```python
from build123d import *

# Parameters (mm, degrees)
F1_DEPTH = 1.5
F2_DEPTH = 14
F4_W     = 30
F4_H     = 17.707149
F5_DEPTH = 26
F6_R     = 3
F7_R     = 1
F9_DEPTH = 21.8


with BuildPart() as f1:
    # F0 (on Top) → F1 (new body)
    with BuildSketch(Plane.XY):
        Polygon((0, -20.207259), (17.5, -10.10363), (17.5, 10.10363), (0, 20.207259), (-17.5, 10.10363), (-17.5, -10.10363), align=None)
        with BuildLine():
            ThreePointArc((-6.29325, -8.626703), (-8.626703, -8.626703), (-8.626703, -6.29325))
            Line((-8.626703, -6.29325), (-6.434672, -4.101219))
            ThreePointArc((-6.434672, -4.101219), (-4.101219, -4.101219), (-4.101219, -6.434672))
            Line((-4.101219, -6.434672), (-6.29325, -8.626703))
        make_face(mode=Mode.SUBTRACT)
        with BuildLine():
            ThreePointArc((8.626703, -6.29325), (8.626703, -8.626703), (6.29325, -8.626703))
            Line((6.29325, -8.626703), (4.101219, -6.434672))
            ThreePointArc((4.101219, -6.434672), (4.101219, -4.101219), (6.434672, -4.101219))
            Line((6.434672, -4.101219), (8.626703, -6.29325))
        make_face(mode=Mode.SUBTRACT)
        with BuildLine():
            ThreePointArc((-8.626703, 6.29325), (-8.626703, 8.626703), (-6.29325, 8.626703))
            Line((-6.29325, 8.626703), (-4.101219, 6.434672))
            ThreePointArc((-4.101219, 6.434672), (-4.101219, 4.101219), (-6.434672, 4.101219))
            Line((-6.434672, 4.101219), (-8.626703, 6.29325))
        make_face(mode=Mode.SUBTRACT)
        with BuildLine():
            Line((4.101219, 6.434672), (6.29325, 8.626703))
            ThreePointArc((6.29325, 8.626703), (8.626703, 8.626703), (8.626703, 6.29325))
            Line((8.626703, 6.29325), (6.434672, 4.101219))
            ThreePointArc((6.434672, 4.101219), (4.101219, 4.101219), (4.101219, 6.434672))
        make_face(mode=Mode.SUBTRACT)
    extrude(amount=F1_DEPTH)

    # F0 (on Top) → F2 (join)
    with BuildSketch(Plane.XY):
        Polygon((-19.9, 11.48927), (-19.9, -11.48927), (0, -22.978541), (19.9, -11.48927), (19.9, 11.48927), (0, 22.978541), align=None)
        Polygon((17.5, 10.10363), (17.5, -10.10363), (0, -20.207259), (-17.5, -10.10363), (-17.5, 10.10363), (0, 20.207259), align=None, mode=Mode.SUBTRACT)
    extrude(amount=F2_DEPTH)

    # F4 (on offset) → F5 (cut)
    with BuildSketch(Plane.XZ.offset(-25)):
        with Locations((0, 10.353574)):
            Rectangle(F4_W, F4_H)
    extrude(amount=F5_DEPTH, mode=Mode.SUBTRACT)

    # F6
    f6_edges = [f1.edges().sort_by_distance(p)[0] for p in [
        (19.9, 11.48927, 7),
        (-19.9, 11.48927, 7),
        (-19.9, -11.48927, 7),
        (0, -22.978541, 7),
        (19.9, -11.48927, 7),
        (17.5, 10.10363, 7.75),
        (17.5, -10.10363, 7.75),
        (0, -20.207259, 7.75),
        (-17.5, -10.10363, 7.75),
        (-17.5, 10.10363, 7.75),
    ]]
    fillet(f6_edges, radius=F6_R)

    # F7
    f7_edges = [f1.edges().sort_by_distance(p)[0] for p in [
        (-15.5, 11.25833, 1.5),
        (0, 22.978541, 0.75),
    ]]
    fillet(f7_edges, radius=F7_R)

    # F8 (on Right) → F9 (cut, symmetric)
    with BuildSketch(Plane.YZ):
        with BuildLine():
            Line((14.684951, 14), (-9.75722, 14))
            add(Edge.make_bspline(
                [(-9.75722, 14), (-1.043614, 14), (10.101545, 12.707566), (14.684951, 5.5)],
                knots=[0, 0, 0, 0, 25.877977, 25.877977, 25.877977, 25.877977], degree=3))
            Line((14.684951, 5.5), (14.684951, 14))
        make_face()
    extrude(amount=F9_DEPTH, both=True, mode=Mode.SUBTRACT)


solid = f1.part
```
Could you check a few things on this model? Use its own coordinates, in mm. A direction names the side the tool comes from. Coordinates: 2 decimals unless noted, no trailing zeros. Order: outer loops, then holes, each group sorted by start corner. A loop starts at its lowest first (then second) coordinate and runs counter-clockwise, first axis right, second up. Notation, with made-up numbers: M -29.5,67 L -6.5,67 A16 ccw -6.5,83 Z; hole C -29,26 d1. An arc over 180 degrees is marked long. Use one line per item in the form item = value. Start each with the question number.
1. We'd pull the mould along X, two halves only. Please class faces 1 (the flat face through (19.9, 0, 7)), 2 (the cylindrical face through (-15.611, 10.865, 1.801)), 3 (the flat face through (-8.648, -15.214, 8.169)), 4 (the cylindrical face through (-19.51, 11.24, 5.13)): +X half, -X half, draft (parallel to the pull), parting line (faces both ways), or undercut.
2. Suppose I cut it at B-B on x = 8. Count the separate pieces of the cut face and the enclosed holes in it, then the cut area to 3 significant figures.
3. On a 3-axis mill with a long thin cutter (end or side, diameter ignored), from which of +Z, -Z, +X, -X, +Y, -Y can I reach the whole of each face in a straight line? I mean faces 5 (the cylindrical face through (19.487, 11.276, 5.126)), 6 (the cylindrical face through (-0.022, -19.743, 8.33)), 7 (the cylindrical face through (17.087, -9.891, 8.33)), 8 (the flat face through (-7.546, -5.213, 0.74)). Say none if no direction works.
4. Suppose I cut it at A-A on z = 1. Write out the boundary of the cut face in (x, y), then the cut area to 3 significant figures.
5. Suppose I cut it at C-C on y = 16.5. Write out the boundary of the cut face in (x, z).
6. For pin 1 (7 mm diameter, centred on x = -2.5, y = 15, fed in from +Z); pin 2 (3 mm diameter, centred on y = 12.5, z = 5, fed in from +X); pin 3 (1 mm diameter, centred on x = 7, z = 12, fed in from -Y), each with a flat end and sliding along its axis, tell me the tip position at first contact or that it passes through.
7. Please list where these lines run through material, in increasing order: line 1 (X direction, y = -8.5, z = 9.5); line 2 (Z direction, x = 14, y = -6.5); line 3 (X direction, y = 10, z = 3.75).
Geometry says:
q1.face_1 = +X half
q1.face_2 = undercut
q1.face_3 = undercut
q1.face_4 = -X half
q2.separate_pieces = 3
q2.enclosed_holes = 0
q2.area = 79.9 mm^2
q3.face_5 = +Z, -Z, +X, +Y
q3.face_6 = +Z, +Y
q3.face_7 = +Z
q3.face_8 = +Z, -Z
q4.outline = M -19.9,-9.76 A3 ccw -18.4,-12.36 L -1.5,-22.11 A3 ccw 1.5,-22.11 L 18.4,-12.36 A3 ccw 19.9,-9.76 L 19.9,9.76 A3 ccw 18.4,12.36 L 0.5,22.69 A1 ccw -0.5,22.69 L -18.4,12.36 A3 ccw -19.9,9.76 Z; hole M -8.63,-6.29 A1.65 ccw -6.29,-8.63 L -4.1,-6.43 A1.65 ccw -6.43,-4.1 Z; hole M -8.63,6.29 L -6.43,4.1 A1.65 ccw -4.1,6.43 L -6.29,8.63 A1.65 ccw Z; hole M 4.1,-6.43 L 6.29,-8.63 A1.65 ccw 8.63,-6.29 L 6.43,-4.1 A1.65 ccw Z; hole M 4.1,6.43 A1.65 ccw 6.43,4.1 L 8.63,6.29 A1.65 ccw 6.29,8.63 Z
q4.area = 1,290 mm^2
q5.outline = M -11.22,0 L 11.22,0 L 11.22,1.5 L -11.22,1.5 Z
q6.pin_1 = 1.5
q6.pin_2 = 19.63
q6.pin_3 = -19.23
q7.line_1 = -19.9 to -17.5, 17.5 to 19.9
q7.line_2 = 0 to 1.5
q7.line_3 = -19.89 to -17.02, 17.02 to 19.89
